```python
from build123d import *

# Parameters (mm, degrees)
PAD_DEPTH       = 20
POCKET_DEPTH    = 30.001
SKETCH002_R     = 4.5
POCKET001_DEPTH = 6
SKETCH003_R     = 3
POCKET002_DEPTH = 15.001
SKETCH004_W     = 15
SKETCH004_H     = 2
POCKET003_DEPTH = 20.001
FILLET_R        = 11


with BuildPart() as part:
    # Sketch → Pad (new body)
    with BuildSketch(Plane.XY):
        with BuildLine():
            Line((-15, -15), (0, -15))
            Line((0, -15), (0, -8))
            ThreePointArc((0, -8), (8, 0), (0, 8))
            Line((0, 15), (0, 8))
            Line((-15, 15), (0, 15))
            Line((-15, 15), (-15, -15))
        make_face()
    extrude(amount=PAD_DEPTH)

    # Sketch001 → Pocket (cut, through all)
    with BuildSketch(Plane(origin=(0, 15, 0), x_dir=(-1, 0, 0), z_dir=(0, 1, 0))):
        with BuildLine():
            Line((19.016133, 20), (19.016133, 0))
            Line((19.016133, 0), (15.335206, 0))
            ThreePointArc((14.016133, 20), (13.069372, 9.894059), (15.335206, 0))
            Line((19.016133, 20), (14.016133, 20))
        make_face()
    extrude(amount=-POCKET_DEPTH, mode=Mode.SUBTRACT)

    # Sketch002 → Pocket001 (cut, symmetric)
    with BuildSketch(Plane.YZ):
        with Locations((10, 10)):
            Circle(SKETCH002_R)
    extrude(amount=POCKET001_DEPTH, both=True, mode=Mode.SUBTRACT)

    # Sketch003 → Pocket002 (cut, through all)
    with BuildSketch(Plane.YZ):
        with Locations((10, 10)):
            Circle(SKETCH003_R)
    extrude(amount=-POCKET002_DEPTH, mode=Mode.SUBTRACT)

    # Sketch004 → Pocket003 (cut, through all)
    with BuildSketch(Plane.XY.offset(20)):
        with Locations((-7.5, -14)):
            Rectangle(SKETCH004_W, SKETCH004_H)
    extrude(amount=-POCKET003_DEPTH, mode=Mode.SUBTRACT)

    # Fillet
    fillet_edges = [part.edges().sort_by_distance(p)[0] for p in [
        (-13.042214, -13, 10.356868),
    ]]
    fillet(fillet_edges, radius=FILLET_R)


solid = part.part
```
Here's how the part is built. I have some questions about the finished solid (model axes, mm). A direction names the side the tool comes from. Give positions to 0.01 mm unless a question says otherwise; leave off trailing zeros. Loops run counter-clockwise (first coordinate to the right, second up) from the corner with the lowest first, then second, coordinate; pieces in that order, holes last. Notation, with made-up numbers: M 34.5,20 L 93.5,20 A6 cw 93.5,30 Z; hole C -9,31 d3. An arc over 180 degrees is marked long. Use one line per item in the form item = value. Start each with the question number.
Q1. If we section it at C-C (y = -7.5): Write out the boundary of the cut face in (x, z), then the cut area to 3 significant figures.
Q2. If we section it at B-B (x = 1.5): Write out the boundary of the cut face in (y, z), then the cut area to 3 significant figures.
Q3. Which directions (+Z, -Z, +X, -X, +Y, -Y) give clear straight access to the entire face, cutting with the end or side of a thin tool? Please do faces 5 (the flat face through (-1, -13, 10)), 6 (the flat face through (-6, 11, 7)), 7 (the flat face through (0, 14.7, 9.9)).
Q4. If we section it at A-A (y = 11): Write out the boundary of the cut face in (x, z).
Q5. Will these pins go through, and if not, where does the flat tip stop? pin 1 Ø1 at (y, z) = (4, 17) entering from +X; pin 2 Ø7 at (y, z) = (9.5, 8) entering from +X; pin 3 Ø2.5 at (y, z) = (-10.5, 13.5) entering from +X; pin 4 Ø5.5 at (y, z) = (10, 10) entering from +X.
Q6. Thinking about a two-plate mould opening in Z: for faces 1 (the flat face through (-6, 1, 20)), 2 (the cylindrical face through (-1.325, 5.504, 10.198)), 3 (the cylindrical face through (-9.64, 12.77, 8.85)), 4 (the flat face through (0, -11, 10)), which applies, +Z half, -Z half, draft (parallel to the pull), parting line (faces both ways), or undercut?
Q7. I need wall thicknesses on line 1 along Z through (x, y) = (-11, 10); line 2 along Y through (x, z) = (-2, 10); line 3 along X through (y, z) = (10, 17). Which ranges of each line are inside material? Lowest first, please.
Q8. If we section it at D-D (y = -0.5): Write out the boundary of the cut face in (x, z), then the cut area to 3 significant figures.
Taken from the geometry:
q1.outline = M -13.75,0 L 2.78,0 L 2.78,20 L -12.5,20 A33.47 cw Z
q1.area = 298 mm^2
q2.outline = M -7.86,0 L 7.86,0 L 7.86,6.04 A4.5 cw 7.86,13.96 L 7.86,20 L -7.86,20 Z
q2.area = 301 mm^2
q3.face_5 = +Z, -Z, +X, -X, -Y
q3.face_6 = +X
q3.face_7 = +Z, -Z, +X, +Y
q4.outline = M -15,0 L 0,0 L 0,5.61 L -6,5.61 L -6,7.17 L -13.37,7.17 A32 cw -15,0.86 Z; M -14.02,20 A32 cw -13.01,12.83 L -6,12.83 L -6,14.39 L 0,14.39 L 0,20 Z
q5.pin_1 = 7.19
q5.pin_2 = 5.29
q5.pin_3 = 0
q5.pin_4 = through
q6.face_1 = +Z half
q6.face_2 = undercut
q6.face_3 = undercut
q6.face_4 = draft
q7.line_1 = 0 to 7, 13 to 20
q7.line_2 = -13 to 5.5, 14.5 to 15
q7.line_3 = -13.39 to 0
q8.outline = M -15,0 L 7.98,0 L 7.98,20 L -14.02,20 A32 cw -15,0.86 Z
q8.area = 431 mm^2
